Build history of the part. All positions in model axes, mm. Face numbers are marked on the shaded views. A direction names the side the tool comes from. Coordinates: 2 decimals unless noted, no trailing zeros. Loops run counter-clockwise (first coordinate to the right, second up) from the corner with the lowest first, then second, coordinate; pieces in that order, holes last.
(1) Slice it at B-B (z = 7.5). Give the cut face in (x, y).
(2) Two-plate mould, pull along Y, no slides. Class the marked faces 1, 2, 3 and 4: pulls with the +Y half, pulls with the -Y half, needs draft (parallel to the pull), parting line crosses it, or undercut.
(3) Flat gauge pins, fed straight in: P1, Ø1.8, axis at x = 0, z = 7.5, coming from the -Y side; P2, Ø1.5, axis at x = 1, y = -3, coming from the +Z side. Where does each tip first touch, or does it go through?
(4) Slice it at A-A (x = 0). Give the cut face in (y, z), and give its area (3 significant figures).
(5) Slice it at C-C (y = -5). Give the cut face in (x, z).
(6) Wall check: L1, parallel to Z at x = 0, y = 0.05; L2, parallel to Z at x = -1.65, y = -2.25; L3, parallel to Y at x = -0.25, z = 5.75. Give the ranges that are in metal, low to high.
(7) Slice it at D-D (z = 4). Give the cut face in (x, y) (1 decimal), and give its area (3 significant figures).
(8) Tool access for the marked faces 5 and 6: list every direction of +Z, -Z, +X, -X, +Y, -Y with a clear straight run to the whole face (end or side of a thin tool).
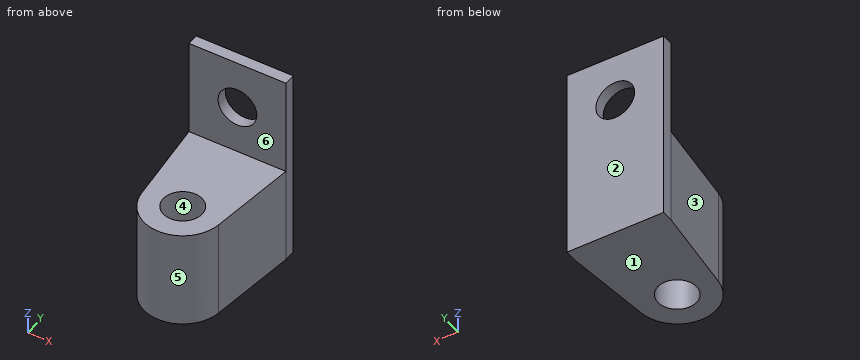
from build123d import *

# Parameters (mm, degrees)
SKETCH2_R           = 0.9975
BOSS_EXTRUDE2_DEPTH = 5
SKETCH3_W           = 5
SKETCH3_H           = 0.593672978
BOSS_EXTRUDE3_DEPTH = 5
SKETCH8_R           = 1
CUT_EXTRUDE2_DEPTH  = 5


with BuildPart() as part:
    # Sketch2 → Boss-Extrude2 (new body)
    with BuildSketch(Plane.XY):
        with BuildLine():
            Line((2.5, -0.161913769), (2.5, 0.431759209))
            Line((2.5, 0.431759209), (-2.5, 0.431759209))
            Line((-2.5, 0.431759209), (-2.5, -0.161913769))
            Line((-2.5, -0.161913769), (-1.987856888, -4.78829759))
            ThreePointArc((-1.987856888, -4.78829759), (0, -6.568240791), (1.987856888, -4.78829759))
            Line((1.987856888, -4.78829759), (2.5, -0.161913769))
        make_face()
        with Locations((0, -4.568240791)):
            Circle(SKETCH2_R, mode=Mode.SUBTRACT)
    extrude(amount=BOSS_EXTRUDE2_DEPTH)

    # Sketch3 → Boss-Extrude3 (add)
    with BuildSketch(Plane.XY.offset(5)):
        with Locations((0, 0.13492272)):
            Rectangle(SKETCH3_W, SKETCH3_H)
    extrude(amount=BOSS_EXTRUDE3_DEPTH)

    # Sketch8 → Cut-Extrude2 (cut)
    with BuildSketch(Plane(origin=(0, -0.161913769, 0), x_dir=(-1, 0, 0), z_dir=(0, -1, 0))):
        with Locations(Location((0, -7.5, 0), (0, 0, 180))):
            Circle(SKETCH8_R)
    extrude(amount=-CUT_EXTRUDE2_DEPTH, mode=Mode.SUBTRACT)


solid = part.part
Response values:
1. outline: (-2.5, -0.16) - (-1, -0.16) - (-1, 0.43) - (-2.5, 0.43) - close; (1, -0.16) - (2.5, -0.16) - (2.5, 0.43) - (1, 0.43) - close
2. face 1: needs draft
2. face 2: pulls with the +Y half
2. face 3: pulls with the -Y half
2. face 4: undercut
3. P1: passes through
3. P2: stops at z = 5
4. outline: (-6.57, 0) - (-5.57, 0) - (-5.57, 5) - (-6.57, 5) - close; (-3.57, 0) - (0.43, 0) - (0.43, 6.5) - (-0.16, 6.5) - (-0.16, 5) - (-3.57, 5) - close; (-0.16, 8.5) - (0.43, 8.5) - (0.43, 10) - (-0.16, 10) - close
4. area: 26.8 mm2
5. outline: (-1.95, 0) - (-0.9, 0) - (-0.9, 5) - (-1.95, 5) - close; (0.9, 0) - (1.95, 0) - (1.95, 5) - (0.9, 5) - close
6. L1: z = 0 to 6.5, 8.5 to 10
6. L2: z = 0 to 5
6. L3: y = -0.16 to 0.43
7. outline: (-2.5, -0.2) - (-2, -4.8) arc R2 ccw to (2, -4.8) - (2.5, -0.2) - (2.5, 0.4) - (-2.5, 0.4) - close; hole circle Ø2 at (0, -4.6)
7. area: 26.0 mm2
8. face 5: +Z, -Z, -Y
8. face 6: +Z, +X, -X, -Y
